Here's how the part is built. I have some questions about the finished solid (model axes, mm). Coordinates: 2 decimals unless noted, no trailing zeros. Write each loop counter-clockwise with the first axis right and the second up, starting at its lowest first coordinate (ties: lowest second). Pieces come first, ordered by that corner, then holes. Notation, with made-up numbers: (-11, 25) -> (1, 25) arc R7 cw to (1, 33) -> close; hole circle Ø11 at (-38, -32). An arc over 180 degrees is marked (long way). Use a Markdown table: item, result. Add a question column.
Item 1: Imagine slicing it at B-B, the plane y = -7.5. Write out the boundary of the cut face in (x, z).
Item 2: Imagine slicing it at A-A, the plane x = 0. Write out the boundary of the cut face in (y, z), and give its area (3 significant figures).
Item 3: If I drill on line 1 along X through (y, z) = (12.5, 2.3); line 2 along Y through (x, z) = (10.5, 2.2); line 3 along X through (y, z) = (32.5, 1), over which ranges is the centre line in solid material (lowest first)? Write a range as from..to.
Item 4: Will this pin go through, and if not, where does the flat tip stop? pin 1 Ø2.5 at (x, y) = (-9.32, 11.39) entering from +Z (3 decimals).
Item 5: If we mould it in two halves opening along Y, with no side actions, what happens to faces 1 (the cylindrical face through (-0.54, -5.06, 1.48)), 2 (the flat face through (1, -52.5, 1)), 3 (the flat face through (-1, 1, 0))? For each: pulls with the +Y half, pulls with the -Y half, needs draft (parallel to the pull), parting line crosses it, or undercut.
Autodesk Inventor part; units mm, degrees
ref_plane "YZ Plane" through (0, 0, 0) normal (1, 0, 0) x (0, 1, 0)
ref_plane "XZ Plane" through (0, 0, 0) normal (0, 1, 0) x (-1, 0, 0)
ref_plane "XY Plane" through (0, 0, 0) normal (0, 0, 1) x (1, 0, 0)
sketch "スケッチ1" plane through (0, 0, 0) normal (0, 0, 1) x (1, 0, 0)
  line L0 (-60, 52.5) -> (60, 52.5)
  line L1 (60, 52.5) -> (60, -52.5)
  line L2 (60, -52.5) -> (-60, -52.5)
  line L3 (-60, -52.5) -> (-60, 52.5)
  line L4 (-60, 52.5) -> (60, -52.5) construction
  line L5 (60, 52.5) -> (-60, -52.5) construction
  line L6 (-105.2334, 22.5) -> (96.2645, 22.5) construction
  circle A0 centre (0, -7.5) radius 2.5
  line L7 (0, 22.5) -> (28.1908, 12.2394) construction
  line L8 (0, 22.5) -> (-28.1908, 12.2394) construction
  line L9 (-9.3204, 11.3924) -> (0, 22.5) construction
  line L10 (9.3204, 33.6076) -> (0, 22.5) construction
  line L11 (0, 85.1475) -> (0, -17.897) construction
  circle A1 centre (-9.3204, 11.3924) radius 2
  circle A2 centre (9.3204, 33.6076) radius 2
  circle A3 centre (28.1908, 12.2394) radius 2.5
  circle A4 centre (-28.1908, 12.2394) radius 2.5
  point P0 (0, 0)
  dimension "d1" = 105
  dimension "d2" = 30
  dimension "d3" = 5
  dimension "d4" = 30
  dimension "d5" = 20
  dimension "d6" = 20
  dimension "d7" = 40
  dimension "d12" = 30
  dimension "d13" = 30
  dimension "d14" = 14.5
  dimension "d15" = 14.5
  dimension "d16" = 4
  dimension "d17" = 4
  dimension "d18" = 5
  dimension "d19" = 5
extrude "押し出し1" add sketch "スケッチ1" along normal blind 3
properties part number "板"
Ans:
| question | item | result |
|---|---|---|
| 1 | outline | (-60, 0) -> (-2.5, 0) -> (-2.5, 3) -> (-60, 3) -> close; (2.5, 0) -> (60, 0) -> (60, 3) -> (2.5, 3) -> close |
| 2 | outline | (-52.5, 0) -> (-10, 0) -> (-10, 3) -> (-52.5, 3) -> close; (-5, 0) -> (52.5, 0) -> (52.5, 3) -> (-5, 3) -> close |
| 2 | area | 300 mm^2 |
| 3 | line 1 | x = -60..-30.68, -25.7..-10.99, -7.66..25.7, 30.68..60 |
| 3 | line 2 | y = -52.5..31.99, 35.22..52.5 |
| 3 | line 3 | x = -60..7.66, 10.99..60 |
| 4 | pin 1 | passes through |
| 5 | face 1 | undercut |
| 5 | face 2 | pulls with the -Y half |
| 5 | face 3 | needs draft |
